Source: CAD feature listing. Evaluate the final solid. Frame: model axes, mm. A direction names the side the tool comes from. Give positions to 0.01 mm unless a question says otherwise; leave off trailing zeros. Loops run counter-clockwise (first coordinate to the right, second up) from the corner with the lowest first, then second, coordinate; pieces in that order, holes last. Notation, with made-up numbers: (32.5, -25.5) - (59.5, -25.5) arc R18 cw to (59.5, 4.5) - close; hole circle Ø3 at (-25, 67.5). An arc over 180 degrees is marked (long way). Put each result on its own line as item: value.
Autodesk Inventor part; units mm, degrees
ref_plane "Work Plane2" through (0, 0, 20.5) normal (0, 0, 1) x (1, 0, 0)
ref_plane "YZ Plane" through (0, 0, 0) normal (1, 0, 0) x (0, 1, 0)
ref_plane "XZ Plane" through (0, 0, 0) normal (0, 1, 0) x (-1, 0, 0)
sketch "Sketch1" plane through (0, 0, 0) normal (0, 0, 1) x (1, 0, 0)
  circle A0 centre (0, 0) radius 20
  circle A1 centre (0, 15.55) radius 1.6
  line L0 (-20, 0) -> (20, 0) construction
  line L1 (20, 0) -> (20, -33)
  line L2 (20, -33) -> (-20, -33)
  line L3 (-20, -33) -> (-20, 0)
  circle A2 centre (-13.4667, 7.775) radius 1.6
  circle A3 centre (-13.4667, -7.775) radius 1.6
  circle A4 centre (0, -15.55) radius 1.6
  circle A5 centre (13.4667, -7.775) radius 1.6
  circle A6 centre (13.4667, 7.775) radius 1.6
  line L4 (0, -7) -> (0, 7) construction
  line L5 (-6.5, -7) -> (-6.5, 7)
  line L6 (6.5, 7) -> (6.5, -7)
  arc A7 (-6.5, -7) -> (6.5, -7) centre (0, -7) ccw
  arc A8 (6.5, 7) -> (-6.5, 7) centre (0, 7) ccw
  dimension "d0" = 40
  dimension "d1" = 15.55
  dimension "d3" = 33
  dimension "d6" = 360
  dimension "d8" = 6.5
  dimension "d9" = 14
extrude "Extrusion1" add sketch "Sketch1" along normal blind 5 contours A0 | L1 L2 L3 A0 | A1 | A2 | A3 | A4 | A5 | A6
sketch "Sketch2" plane through (0, 0, 0) normal (0, 0, -1) x (-1, 0, 0)
  line L0 (20, 0) -> (20, -33)
  arc A0 (20, 0) -> (-20, 0) centre (0, 0) ccw
  line L1 (-20, -33) -> (-20, 0)
  line L2 (20, -33) -> (-20, -33)
  line L3 (-6.5, 7) -> (-6.5, -7)
  arc A1 (6.5, 7) -> (-6.5, 7) centre (0, 7) ccw
  line L4 (6.5, -7) -> (6.5, 7)
  arc A2 (-6.5, -7) -> (6.5, -7) centre (0, -7) ccw
  circle A3 centre (0, 0) radius 15.5 construction
  circle A4 centre (-7.75, 13.4234) radius 1.6
  line L5 (0, 0) -> (-7.75, 13.4234) construction
  line L6 (0, 0) -> (0, 15.5) construction
  circle A5 centre (-15.5, 0) radius 1.6
  circle A6 centre (-7.75, -13.4234) radius 1.6
  circle A7 centre (7.75, -13.4234) radius 1.6
  circle A8 centre (15.5, 0) radius 1.6
  circle A9 centre (7.75, 13.4234) radius 1.6
  dimension "d12" = 31
  dimension "d13" = 3.2
  dimension "d14" = 30
  dimension "d17" = 360
extrude "Extrusion2" cut sketch "Sketch2" against normal blind 5 contours A4 | A5 | A6 | A7 | A8 | A9
sketch "Sketch3" plane through (-20, -33, 0) normal (0, -1, 0) x (1, 0, 0)
  line L0 (0, 0) -> (40, 0)
  line L1 (40, 0) -> (40, 5)
  line L2 (0, 5) -> (40, 5)
  line L3 (0, 0) -> (0, 5)
  line L4 (40, 0) -> (40, 5)
  line L5 (40, 5) -> (0, 5)
  line L6 (0, 5) -> (0, 40)
  line L7 (0, 40) -> (40, 40)
  line L8 (40, 40) -> (40, 5)
  point P0 (20, 0)
  dimension "d21" = 40
extrude "Extrusion3" add sketch "Sketch3" against normal blind 8 contours L6 L7 L8 L2
fillet "Fillet1" radius 2 1 edges at (0, -33, 0)
sketch "Sketch4" plane through (-20, -33, 2) normal (0, -1, 0) x (1, 0, 0)
  line L0 (40, 38) -> (0, 38)
  line L1 (0, 0) -> (0, 38)
  line L2 (40, 0) -> (0, 0)
  line L3 (40, 0) -> (40, 38)
  line L4 (5, 4) -> (-5, 4)
  line L5 (-5, 4) -> (-5, 11)
  line L6 (-5, 11) -> (5, 11)
  line L7 (5, 11) -> (5, 4)
  line L8 (5, 4) -> (-5, 11) construction
  line L9 (-5, 4) -> (5, 11) construction
  circle A0 centre (-5, 7.5) radius 3.5
  circle A1 centre (-5, 7.5) radius 1.75
  point P0 (20, -2)
  point P1 (0, 7.5)
  point P2 (0, 4)
  point P3 (0, 11)
  point P4 (-5, 11)
  dimension "d26" = 7
  dimension "d27" = 5
  dimension "d28" = 4
  dimension "d29" = 3.5
extrude "Extrusion4" add sketch "Sketch4" against normal blind 4 contours L1 L4 A0 L6 | A0 L5 A1 | L5 A1 A0
ref_plane "Work Plane1" through (0, 0, 22.5) normal (0, 0, 1) x (1, 0, 0)
ref_plane "Work Plane2" through (0, 0, 20.5) normal (0, 0, 1) x (1, 0, 0)
mirror "Mirror2" about plane through (0, 0, 0) normal (1, 0, 0) of "Extrusion4"
mirror "Mirror3" about plane through (0, 0, 20.5) normal (0, 0, 1) of "Extrusion4", "Mirror2"
fillet "Fillet4" radius 2 8 edges at (20, -31, 6) (20, -31, 28) (-20, -31, 6) (-20, -31, 13) (-20, -31, 28) (-20, -31, 35) (20, -31, 35) (20, -31, 13)
properties part number "08_Ga_dong_co" material "Polyethylene, High Density"
1) Section query A-A, the plane x = 0. Output: boundary loops of the cut face in (y, z), plus the area to 3 significant figures.
Check result:
outline: (-33, 2) arc R2 ccw to (-31, 0) - (-13.5, 0) - (-13.5, 5) - (-25, 5) - (-25, 40) - (-33, 40) - close; (13.5, 0) - (20, 0) - (20, 5) - (13.5, 5) - close
area: 409 mm²
2) Material intervals for line 1 along X through (y, z) = (-30.35, 31.5); line 2 along Z through (x, y) = (25, -31.65); line 3 along Y through (x, z) = (7.75, 1.85), sorted ascending. Write a range as [from, to].
Check result:
line 1: [-28.5, -26.75], [-23.25, 23.25], [26.75, 28.5]
line 2: [6, 7.75], [11.25, 13], [28, 29.75], [33.25, 35]
line 3: [-32.99, -15.02], [-11.82, 11.82], [15.02, 18.44]
3) Pin query (flat end, axial travel): P1, Ø2.5, axis at x = 23.5, y = -31.5, coming from the +Z side; P2, Ø3.5, axis at x = 23.5, y = -30, coming from the -Z side; P3, Ø6, axis at x = 10.5, z = 32, coming from the +Y side. Return the tip coordinate at first contact, or that it passes through.
Check result:
P1: z = 35
P2: z = 5.98
P3: y = -25
4) Section query B-B, the plane y = -6. Output: boundary loops of the cut face in (x, z).
Check result:
outline: (-20, 0) - (-6.5, 0) - (-6.5, 5) - (-20, 5) - close; (6.5, 0) - (20, 0) - (20, 5) - (6.5, 5) - close
5) Section query D-D, the plane z = 14. Output: boundary loops of the cut face in (x, y).
Check result:
outline: (-20.27, -33) - (20.27, -33) - (20.27, -29) - (20, -29) - (20, -25) - (-20, -25) - (-20, -29) - (-20.27, -29) - close
6) Access query for faces 4 (the flat face through (-23, -31, 28)), 5 (the flat face through (-23, -31, 6)), 6 (the flat face through (-5, -12, 5)), 7 (the flat face through (6.5, 0, 2)), 8 (the flat face through (23, -29, 10)). Directions: +Z, -Z, +X, -X, +Y, -Y. A direction counts if a zero-diameter tool reaches every point of the face in a straight line with its end or side. Return the directions, or none.
Check result:
face 4: -X, +Y, -Y
face 5: -Z, -X, +Y, -Y
face 6: +Z, +X, -X, +Y
face 7: +Z, -Z
face 8: +Z, -Z, +X, +Y
7) Mould query, pull axis Z, two halves, no side actions, for faces 1 (the flat face through (-23, -29, 11)), 2 (the cylindrical face through (26.75, -31.03, 9.42)), 3 (the flat face through (24, -31, 6)). Classes: pulls with the +Z half, pulls with the -Z half, needs draft (parallel to the pull), parting line crosses it, or undercut.
Check result:
face 1: needs draft
face 2: undercut
face 3: pulls with the -Z half
8) Section query C-C, the plane x = -7.75. Output: boundary loops of the cut face in (y, z).
Check result:
outline: (-33, 2) arc R2 ccw to (-31, 0) - (-15.02, 0) - (-15.02, 5) - (-25, 5) - (-25, 40) - (-33, 40) - close; (-11.82, 0) - (11.82, 0) - (11.82, 5) - (-11.82, 5) - close; (15.02, 0) - (18.44, 0) - (18.44, 5) - (15.02, 5) - close
